from build123d import *
from build123d.topology import SkipClean

# Parameters (mm, degrees)
SKETCH1_R                = 9.5
BOSS_EXTRUDE1_DEPTH      = 48
SKETCH2_W                = 34
SKETCH2_H                = 30
CUT_EXTRUDE1_DEPTH       = 62.481704596
BOSS_EXTRUDE2_START      = -2.5
SKETCH3_R                = 9.5
SKETCH3_R_2              = 2.4
BOSS_EXTRUDE2_DEPTH      = 2.5
SKETCH4_R                = 9.5
SKETCH4_R_2              = 4.2
BOSS_EXTRUDE3_DEPTH      = 7
SKETCH5_R                = 4.2
BOSS_EXTRUDE4_DEPTH      = 11
BOSS_EXTRUDE5_DEPTH      = 48
CUT_EXTRUDE2_START       = -48
CUT_EXTRUDE2_OUTLINE_R   = 2.65
CUT_EXTRUDE2_DEPTH       = 48
CUT_EXTRUDE3_START       = -4.5
SKETCH8_R                = 9.5
CUT_EXTRUDE3_DEPTH       = 4.5
SKETCH9_R                = 6.067807638
CUT_EXTRUDE4_DEPTH       = 4.5
SKETCH10_R               = 9.5
BOSS_EXTRUDE6_DEPTH      = 4.5
SKETCH11_R               = 4.2
BOSS_EXTRUDE7_DEPTH      = 3.5
SKETCH12_R               = 2.4
BOSS_EXTRUDE8_DEPTH      = 2.5
SKETCH13_W               = 35
SKETCH13_H               = 34
CUT_EXTRUDE5_DEPTH       = 14.5
SKETCH15_R               = 3.436413098
BOSS_EXTRUDE9_DEPTH      = 10
BOSS_EXTRUDE10_DEPTH     = 0.5
SKETCH18_R               = 4.2
CUT_EXTRUDE8_DEPTH       = 0.5
CUT_EXTRUDE9_DEPTH       = 69.529190861
BOSS_EXTRUDE11_DEPTH     = 7
CUT_EXTRUDE10_DEPTH      = 80.22909819
BOSS_EXTRUDE12_DEPTH     = 41.5
SKETCH25_R               = 4.2
CUT_EXTRUDE11_DEPTH      = 0.5
CUT_EXTRUDE12_DEPTH      = 80.22909819
CUT_EXTRUDE12_DEPTH_BACK = 80.22909819


# Read off the part's stored shape, not the designer's step: Cut-Extrude2
with BuildPart() as part:
    # Sketch1 → Boss-Extrude1 (new body)
    with BuildSketch(Plane.XY):
        with BuildLine():
            Line((-12, 0), (-12, 30))
            Line((-12, 30), (12, 30))
            Line((12, 30), (12, 0))
            ThreePointArc((12, 0), (0, -12), (-12, 0))
        make_face()
        Circle(SKETCH1_R, mode=Mode.SUBTRACT)
    extrude(amount=-BOSS_EXTRUDE1_DEPTH)

    # Sketch2 → Cut-Extrude1 (cut, through all)
    with BuildSketch(Plane.ZY.offset(12)):
        with Locations((-24, 3)):
            Rectangle(SKETCH2_W, SKETCH2_H)
    extrude(amount=-CUT_EXTRUDE1_DEPTH, mode=Mode.SUBTRACT)

    # Sketch3 → Boss-Extrude2 (add)
    with BuildSketch(Plane(origin=(0, 0, -48), x_dir=(-1, 0, 0), z_dir=(0, 0, -1)).offset(BOSS_EXTRUDE2_START)):
        Circle(SKETCH3_R)
        Circle(SKETCH3_R_2, mode=Mode.SUBTRACT)
    extrude(amount=BOSS_EXTRUDE2_DEPTH)

    # Sketch4 → Boss-Extrude3 (add)
    with BuildSketch(Plane.XY):
        with Locations(Location((0, 0, 0), (0, 0, 180))):
            Circle(SKETCH4_R)
        Circle(SKETCH4_R_2, mode=Mode.SUBTRACT)
    extrude(amount=-BOSS_EXTRUDE3_DEPTH)

    # Sketch5 → Boss-Extrude4 (add)
    with BuildSketch(Plane.XY):
        Circle(SKETCH5_R)
    extrude(amount=-BOSS_EXTRUDE4_DEPTH)

    # Sketch6 → Boss-Extrude5 (add)
    with BuildSketch(Plane(origin=(0, 0, -48), x_dir=(-1, 0, 0), z_dir=(0, 0, -1))):
        Polygon((12, 30), (12, 18), (18, 18), (38, 18), (38, 30), align=None)
    extrude(amount=-BOSS_EXTRUDE5_DEPTH)

    # Cut-Extrude2 outline → Cut-Extrude2 (cut)
    with BuildSketch(Plane.XY.offset(CUT_EXTRUDE2_START)):
        Circle(CUT_EXTRUDE2_OUTLINE_R)
    extrude(amount=CUT_EXTRUDE2_DEPTH, mode=Mode.SUBTRACT)

    # Sketch8 → Cut-Extrude3 (cut)
    with BuildSketch(Plane(origin=(0, 0, -7), x_dir=(-1, 0, 0), z_dir=(0, 0, -1)).offset(CUT_EXTRUDE3_START)):
        Circle(SKETCH8_R)
    extrude(amount=CUT_EXTRUDE3_DEPTH, mode=Mode.SUBTRACT)


with BuildPart() as cut_extrude3_piece_1:
    # of the separate pieces the step leaves, piece 1, a body of its own (cut_extrude3_pieces)
    add(part.part.solids().sort_by_distance((-12, 0, 0))[0])

    # Sketch10 → Boss-Extrude6 (add)
    with BuildSketch(Plane.XY.offset(-45.5)):
        with Locations(Location((0, 0, 0), (0, 0, 90))):
            Circle(SKETCH10_R)
    extrude(amount=BOSS_EXTRUDE6_DEPTH)

    # Sketch11 → Boss-Extrude7 (add)
    with BuildSketch(Plane.XY.offset(-41)):
        with Locations(Location((0, 0, 0), (0, 0, 180))):
            Circle(SKETCH11_R)
    extrude(amount=BOSS_EXTRUDE7_DEPTH)

    # Sketch12 → Boss-Extrude8 (add)
    with BuildSketch(Plane(origin=(0, 0, -48), x_dir=(-1, 0, 0), z_dir=(0, 0, -1))):
        Circle(SKETCH12_R)
    extrude(amount=-BOSS_EXTRUDE8_DEPTH)

    # Sketch13 → Cut-Extrude5 (cut)
    with BuildSketch(Plane(origin=(0, 30, 0), x_dir=(1, 0, 0), z_dir=(0, 1, 0))):
        with Locations((-5.5, 24)):
            Rectangle(SKETCH13_W, SKETCH13_H)
    extrude(amount=-CUT_EXTRUDE5_DEPTH, mode=Mode.SUBTRACT)

    # Sketch15 → Boss-Extrude9 (add)
    with BuildSketch(Plane(origin=(0, 0, -48), x_dir=(-1, 0, 0), z_dir=(0, 0, -1))):
        Circle(SKETCH15_R)
    extrude(amount=-BOSS_EXTRUDE9_DEPTH)

    # Sketch16 → Boss-Extrude10 (add)
    with SkipClean():  # the faces are left unmerged after this step: merging them gives an invalid solid
        with BuildSketch(Plane(origin=(0, 0, -48), x_dir=(-1, 0, 0), z_dir=(0, 0, -1))):
            Polygon((38, 30), (-12, 30), (-12, 18), (12, 18), (38, 18), align=None)
            with BuildLine():
                Line((-12, 0), (12, 0))
                ThreePointArc((12, 0), (0, -12), (-12, 0))
            make_face()
            with BuildLine():
                ThreePointArc((12, 0), (0, 12), (-12, 0))
                Line((-12, 0), (12, 0))
            make_face()
            with BuildLine():
                Line((12, 0), (-12, 0))
                ThreePointArc((-12, 0), (0, -12), (12, 0))
            make_face()
            with BuildLine():
                Line((12, 18), (-12, 18))
                Line((-12, 18), (-12, 0))
                ThreePointArc((-12, 0), (0, 12), (12, 0))
                Line((12, 0), (12, 18))
            make_face()
        extrude(amount=BOSS_EXTRUDE10_DEPTH)

    # Sketch18 → Cut-Extrude8 (cut)
    with SkipClean():  # the faces are left unmerged after this step: merging them gives an invalid solid
        with BuildSketch(Plane.XY.offset(-41)):
            with BuildLine():
                Line((12, 30), (-23, 30))
                Line((-23, 30), (-23, 18))
                Line((-23, 18), (-12, 18))
                Line((-12, 18), (-12, 0))
                ThreePointArc((-12, 0), (0, -12), (12, 0))
                Line((12, 0), (12, 30))
            make_face()
            Circle(SKETCH18_R, mode=Mode.SUBTRACT)
        extrude(amount=-CUT_EXTRUDE8_DEPTH, mode=Mode.SUBTRACT)

    # Sketch19 → Cut-Extrude9 (cut, through all)
    with SkipClean():  # the faces are left unmerged after this step: merging them gives an invalid solid
        with BuildSketch(Plane.XY):
            with BuildLine():
                ThreePointArc((11, 0), (0, -11), (-11, 0))
                Line((-11, 0), (-12, 0))
                ThreePointArc((-12, 0), (0, -12), (12, 0))
                Line((12, 0), (12, 30))
                Line((12, 30), (11, 30))
                Line((11, 30), (11, 0))
            make_face()
        extrude(amount=-CUT_EXTRUDE9_DEPTH, mode=Mode.SUBTRACT)

    # Sketch21 → Boss-Extrude11 (add)
    with SkipClean():  # the faces are left unmerged after this step: merging them gives an invalid solid
        with BuildSketch(Plane.XY):
            with BuildLine():
                Line((-55, -11), (0, -11))
                ThreePointArc((0, -11), (-7.778174593, -7.778174593), (-11, 0))
                Line((-11, 0), (-12, 0))
                Line((-12, 0), (-12, 18))
                Line((-12, 18), (-29.285566016, 18))
                ThreePointArc((-29.285566016, 18), (-44.085437149, 5.222560402), (-55, -11))
            make_face()
        boss_extrude11 = extrude(amount=-BOSS_EXTRUDE11_DEPTH)

    # Mirror2: Boss-Extrude11 across plane
    with SkipClean():  # the faces are left unmerged after this step: merging them gives an invalid solid
        add(boss_extrude11.mirror(Plane.XY.offset(-24.25)))

    # Sketch23 → Cut-Extrude10 (cut, through all)
    with SkipClean():  # the faces are left unmerged after this step: merging them gives an invalid solid
        with BuildSketch(Plane.XY):
            with BuildLine():
                Line((11, 30), (-38, 30))
                Line((-38, 30), (-38, 11.325220695))
                ThreePointArc((-38, 11.325220695), (-15.219016868, 25.173069355), (11, 30))
            make_face()
        extrude(amount=-CUT_EXTRUDE10_DEPTH, mode=Mode.SUBTRACT)

    # Sketch24 → Boss-Extrude12 (add)
    with SkipClean():  # the faces are left unmerged after this step: merging them gives an invalid solid
        with BuildSketch(Plane.XY):
            with BuildLine():
                ThreePointArc((-23, 21.6788275), (-41.60205739, 7.887419381), (-55, -11))
                Line((-55, -11), (-51.635998377, -11))
                ThreePointArc((-51.635998377, -11), (-39.486754135, 5.75970176), (-23, 18.276837089))
                Line((-23, 18.276837089), (-23, 21.6788275))
            make_face()
        extrude(amount=-BOSS_EXTRUDE12_DEPTH)

    # Sketch25 → Cut-Extrude11 (cut)
    # profile 1 of 3: a face of its own
    with BuildSketch(Plane.XY.offset(-41.5)):
        with BuildLine():
            ThreePointArc((11, 27), (-6.550595226, 24.784456384), (-23, 18.276837089))
            Line((-23, 18.276837089), (-23, 18))
            Line((-23, 18), (-23.499204657, 18))
            ThreePointArc((-23.499204657, 18), (-39.685914386, 5.555259732), (-51.635998377, -11))
            Line((-51.635998377, -11), (0, -11))
            ThreePointArc((0, -11), (-7.778174593, 7.778174593), (11, 0))
            Line((11, 0), (11, 27))
        make_face()
    # profile 2 of 3: a face of its own
    with BuildSketch(Plane.XY.offset(-41.5)):
        with BuildLine():
            ThreePointArc((0, -11), (7.778174593, -7.778174593), (11, 0))
            ThreePointArc((11, 0), (-7.778174593, 7.778174593), (0, -11))
        make_face()
        Circle(SKETCH25_R, mode=Mode.SUBTRACT)
    # profile 3 of 3: a face of its own
    with BuildSketch(Plane.XY.offset(-41.5)):
        with BuildLine():
            ThreePointArc((11, 30), (-6.501727856, 27.889455027), (-23, 21.6788275))
            Line((-23, 21.6788275), (-23, 18.276837089))
            ThreePointArc((-23, 18.276837089), (-6.550595226, 24.784456384), (11, 27))
            Line((11, 27), (11, 30))
        make_face()
    extrude(amount=-CUT_EXTRUDE11_DEPTH, mode=Mode.SUBTRACT)

    # Sketch26 → Cut-Extrude12 (cut, two sides: drawn at the far end of the back side and taken through both)
    with BuildSketch(Plane(origin=(0, 0, -48.5), x_dir=(-1, 0, 0), z_dir=(0, 0, -1)).offset(-CUT_EXTRUDE12_DEPTH_BACK)):
        with BuildLine():
            Line((15, -11), (15, 4))
            Line((15, 4), (21.056677648, 13.637195648))
            ThreePointArc((21.056677648, 13.637195648), (32.64899906, 7.412367977), (42.766432542, -1))
            Line((42.766432542, -1), (55, -1))
            Line((55, -1), (55, -11))
            Line((55, -11), (15, -11))
        make_face()
    extrude(amount=CUT_EXTRUDE12_DEPTH + CUT_EXTRUDE12_DEPTH_BACK, mode=Mode.SUBTRACT)


with BuildPart() as cut_extrude3_piece_2:
    # of the separate pieces the step leaves, piece 2, a body of its own (cut_extrude3_pieces)
    add(part.part.solids().sort_by_distance((4.2, 0, -7))[0])

    # Sketch9 → Cut-Extrude4 (cut)
    with BuildSketch(Plane(origin=(0, 0, -11), x_dir=(-1, 0, 0), z_dir=(0, 0, -1))):
        Circle(SKETCH9_R)
    extrude(amount=-CUT_EXTRUDE4_DEPTH, mode=Mode.SUBTRACT)


solid = cut_extrude3_piece_1.part
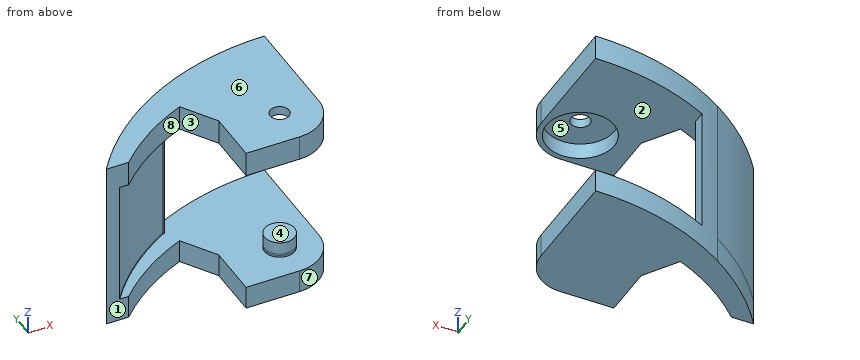
The listing builds one solid part. Answer for the finished solid, in the listing's coordinates (mm). Face numbers are marked on the shaded views. A direction names the side the tool comes from. Round coordinates to 2 decimals unless told otherwise and drop trailing zeros. Write each loop counter-clockwise with the first axis right and the second up, starting at its lowest first coordinate (ties: lowest second). Pieces come first, ordered by that corner, then holes. Notation, with made-up numbers: M 4.25,76.5 L 29.25,76.5 A33 cw 29.25,115.5 Z; hole C -11.75,16.5 d11. An arc over 180 degrees is marked long. Write each question's results on one line, items separated by ' | '. Start each with the question number.
(1) The part is cut by section A-A, the plane y = 26. Write down the section's boundary in (x, z).
(2) The part is cut by section C-C, the plane z = -43.5. Write down the section's boundary in (x, y).
(3) The part is cut by section D-D, the plane y = 8. Write down the section's boundary in (x, z).
(4) Determine the mould class of the marked faces 6, 7 and 8 for opening direction X: +X half, -X half, draft (parallel to the pull), parting line (faces both ways), or undercut.
(5) Find the intervals of material crossed by line 1 (Z direction, x = -2, y = 7); line 2 (Z direction, x = 6.5, y = 20.5); line 3 (X direction, y = 0, z = -1.6), in increasing order.
(6) The part is cut by section B-B, the plane x = -16. Write down the section's boundary in (y, z), and give its area (3 significant figures).
(7) Each of these flat-tipped pins is pushed along its axis until it touches: P1, Ø1.1, axis at y = 20.5, z = -17.5, coming from the +X side; P2, Ø5, axis at x = -40, z = -40.5, coming from the -Y side; P3, Ø3, axis at y = -6.5, z = -44, coming from the -X side. Where does it stop, or does it pass through?
(8) For the marked faces 1, 2, 3, 4 and 5, determine the directions among +Z, -Z, +X, -X, +Y, -Y from which every point of the face is accessible in a straight line to the end or side of a thin tool.
Worked answers:
1) outline: M -12.94,-48.5 L 11,-48.5 L 11,-42 L -12.94,-42 Z; M -12.94,-7 L 11,-7 L 11,0 L -12.94,0 Z
2) outline: M -49.03,-1 L -42.77,-1 A65.62 cw -21.06,13.64 L -15,4 L -15,-11 L 0,-11 A11 ccw 11,0 L 11,30 A73.62 ccw Z
3) outline: M -41.49,-48.5 L -31.76,-48.5 L -31.76,-42 L -37.19,-42 L -37.19,-7 L -31.76,-7 L -31.76,0 L -41.49,0 Z; M -17.51,-48.5 L 11,-48.5 L 11,-42 L -17.51,-42 Z; M -17.51,-7 L -5.12,-7 L -5.12,-2.5 L 5.12,-2.5 L 5.12,-7 L 11,-7 L 11,0 L -17.51,0 Z
4) face 6: draft | face 7: +X half | face 8: undercut
5) line 1: z = -48.5 to -42, -2.5 to 0 | line 2: z = -48.5 to -42, -7 to 0 | line 3: x = -48.31 to -41.76, -15 to -2.65, 2.65 to 11
6) outline: M 5.59,-48.5 L 24.87,-48.5 L 24.87,-42 L 5.59,-42 Z; M 5.59,-7 L 24.87,-7 L 24.87,0 L 5.59,0 Z | area: 260 mm²
7) P1: stops at x = -23 | P2: stops at y = -0.23 | P3: stops at x = -15
8) face 1: +Z, -Z, -X, -Y | face 2: +X, -Y | face 3: +Z, -Z, -Y | face 4: +X, +Y, -Y | face 5: none
